Part model, mm, in its own coordinate system. Face numbers are marked on the shaded views. A direction names the side the tool comes from. Give positions to 0.01 mm unless a question says otherwise; leave off trailing zeros. Order: outer loops, then holes, each group sorted by start corner. A loop starts at its lowest first (then second) coordinate and runs counter-clockwise, first axis right, second up.
from build123d import *

# Parameters (mm, degrees)
SKETCH_7_W          = 180
SKETCH_7_H          = 128
EXTRUDE_1_DEPTH     = 2300
SKETCH_8_R          = 11.5
CUT_EXTRUDE_1_DEPTH = 16
SKETCH_9_R          = 11.5
CUT_EXTRUDE_2_DEPTH = 16


with BuildPart() as part:
    # 草图7 → 凸台-拉伸1 (new body)
    with BuildSketch(Plane(origin=(0, 0, 0), x_dir=(0, 0, -1), z_dir=(1, 0, 0))):
        Polygon((-315, 16), (-315, 0), (315, 0), (315, 16), (106, 16), (106, 144), (150, 144), (150, 160), (-150, 160), (-150, 144), (-106, 144), (-106, 16), align=None)
        with Locations((0, 80)):
            Rectangle(SKETCH_7_W, SKETCH_7_H, mode=Mode.SUBTRACT)
    extrude(amount=EXTRUDE_1_DEPTH)

    # 草图8 → 切除-拉伸1 (cut)
    with BuildSketch(Plane(origin=(0, 160, 0), x_dir=(1, 0, 0), z_dir=(0, 1, 0))):
        with Locations(Location((462.5, 62.5, 0), (0, 0, 270))):
            Circle(SKETCH_8_R)
        with Locations(Location((587.5, 62.5, 0), (0, 0, 270))):
            Circle(SKETCH_8_R)
        with Locations(Location((462.5, -62.5, 0), (0, 0, 270))):
            Circle(SKETCH_8_R)
        with Locations(Location((587.5, -62.5, 0), (0, 0, 270))):
            Circle(SKETCH_8_R)
        with Locations(Location((1712.5, 62.5, 0), (0, 0, 270))):
            Circle(SKETCH_8_R)
        with Locations(Location((1837.5, 62.5, 0), (0, 0, 270))):
            Circle(SKETCH_8_R)
        with Locations(Location((1712.5, -62.5, 0), (0, 0, 270))):
            Circle(SKETCH_8_R)
        with Locations(Location((1837.5, -62.5, 0), (0, 0, 270))):
            Circle(SKETCH_8_R)
    extrude(amount=-CUT_EXTRUDE_1_DEPTH, mode=Mode.SUBTRACT)

    # 草图9 → 切除-拉伸2 (cut)
    with BuildSketch(Plane.XZ):
        with Locations(Location((110, 260, 0), (0, 0, 270))):
            Circle(SKETCH_9_R)
        with Locations(Location((190, 260, 0), (0, 0, 270))):
            Circle(SKETCH_9_R)
        with Locations(Location((410, 260, 0), (0, 0, 270))):
            Circle(SKETCH_9_R)
        with Locations(Location((490, 260, 0), (0, 0, 270))):
            Circle(SKETCH_9_R)
        with Locations(Location((710, 260, 0), (0, 0, 270))):
            Circle(SKETCH_9_R)
        with Locations(Location((790, 260, 0), (0, 0, 270))):
            Circle(SKETCH_9_R)
        with Locations(Location((1110, 260, 0), (0, 0, 270))):
            Circle(SKETCH_9_R)
        with Locations(Location((1190, 260, 0), (0, 0, 270))):
            Circle(SKETCH_9_R)
        with Locations(Location((1510, 260, 0), (0, 0, 270))):
            Circle(SKETCH_9_R)
        with Locations(Location((1590, 260, 0), (0, 0, 270))):
            Circle(SKETCH_9_R)
        with Locations(Location((1810, 260, 0), (0, 0, 270))):
            Circle(SKETCH_9_R)
        with Locations(Location((1890, 260, 0), (0, 0, 270))):
            Circle(SKETCH_9_R)
        with Locations(Location((110, 180, 0), (0, 0, 270))):
            Circle(SKETCH_9_R)
        with Locations(Location((190, 180, 0), (0, 0, 270))):
            Circle(SKETCH_9_R)
        with Locations(Location((410, 180, 0), (0, 0, 270))):
            Circle(SKETCH_9_R)
        with Locations(Location((490, 180, 0), (0, 0, 270))):
            Circle(SKETCH_9_R)
        with Locations(Location((710, 180, 0), (0, 0, 270))):
            Circle(SKETCH_9_R)
        with Locations(Location((790, 180, 0), (0, 0, 270))):
            Circle(SKETCH_9_R)
        with Locations(Location((1110, 180, 0), (0, 0, 270))):
            Circle(SKETCH_9_R)
        with Locations(Location((1190, 180, 0), (0, 0, 270))):
            Circle(SKETCH_9_R)
        with Locations(Location((1510, 180, 0), (0, 0, 270))):
            Circle(SKETCH_9_R)
        with Locations(Location((1590, 180, 0), (0, 0, 270))):
            Circle(SKETCH_9_R)
        with Locations(Location((1810, 180, 0), (0, 0, 270))):
            Circle(SKETCH_9_R)
        with Locations(Location((1890, 180, 0), (0, 0, 270))):
            Circle(SKETCH_9_R)
        with Locations(Location((110, -140, 0), (0, 0, 270))):
            Circle(SKETCH_9_R)
        with Locations(Location((190, -140, 0), (0, 0, 270))):
            Circle(SKETCH_9_R)
        with Locations(Location((410, -140, 0), (0, 0, 270))):
            Circle(SKETCH_9_R)
        with Locations(Location((490, -140, 0), (0, 0, 270))):
            Circle(SKETCH_9_R)
        with Locations(Location((710, -140, 0), (0, 0, 270))):
            Circle(SKETCH_9_R)
        with Locations(Location((790, -140, 0), (0, 0, 270))):
            Circle(SKETCH_9_R)
        with Locations(Location((1110, -140, 0), (0, 0, 270))):
            Circle(SKETCH_9_R)
        with Locations(Location((1190, -140, 0), (0, 0, 270))):
            Circle(SKETCH_9_R)
        with Locations(Location((1510, -140, 0), (0, 0, 270))):
            Circle(SKETCH_9_R)
        with Locations(Location((1590, -140, 0), (0, 0, 270))):
            Circle(SKETCH_9_R)
        with Locations(Location((1810, -140, 0), (0, 0, 270))):
            Circle(SKETCH_9_R)
        with Locations(Location((1890, -140, 0), (0, 0, 270))):
            Circle(SKETCH_9_R)
        with Locations(Location((110, -220, 0), (0, 0, 270))):
            Circle(SKETCH_9_R)
        with Locations(Location((190, -220, 0), (0, 0, 270))):
            Circle(SKETCH_9_R)
        with Locations(Location((410, -220, 0), (0, 0, 270))):
            Circle(SKETCH_9_R)
        with Locations(Location((490, -220, 0), (0, 0, 270))):
            Circle(SKETCH_9_R)
        with Locations(Location((710, -220, 0), (0, 0, 270))):
            Circle(SKETCH_9_R)
        with Locations(Location((790, -220, 0), (0, 0, 270))):
            Circle(SKETCH_9_R)
        with Locations(Location((1110, -220, 0), (0, 0, 270))):
            Circle(SKETCH_9_R)
        with Locations(Location((1190, -220, 0), (0, 0, 270))):
            Circle(SKETCH_9_R)
        with Locations(Location((1510, -220, 0), (0, 0, 270))):
            Circle(SKETCH_9_R)
        with Locations(Location((1590, -220, 0), (0, 0, 270))):
            Circle(SKETCH_9_R)
        with Locations(Location((1810, -220, 0), (0, 0, 270))):
            Circle(SKETCH_9_R)
        with Locations(Location((1890, -220, 0), (0, 0, 270))):
            Circle(SKETCH_9_R)
        with Locations(Location((2110, 260, 0), (0, 0, 270))):
            Circle(SKETCH_9_R)
        with Locations(Location((2190, 260, 0), (0, 0, 270))):
            Circle(SKETCH_9_R)
        with Locations(Location((2110, 180, 0), (0, 0, 270))):
            Circle(SKETCH_9_R)
        with Locations(Location((2190, 180, 0), (0, 0, 270))):
            Circle(SKETCH_9_R)
        with Locations(Location((2110, -140, 0), (0, 0, 270))):
            Circle(SKETCH_9_R)
        with Locations(Location((2190, -140, 0), (0, 0, 270))):
            Circle(SKETCH_9_R)
        with Locations(Location((2110, -220, 0), (0, 0, 270))):
            Circle(SKETCH_9_R)
        with Locations(Location((2190, -220, 0), (0, 0, 270))):
            Circle(SKETCH_9_R)
    extrude(amount=-CUT_EXTRUDE_2_DEPTH, mode=Mode.SUBTRACT)


solid = part.part
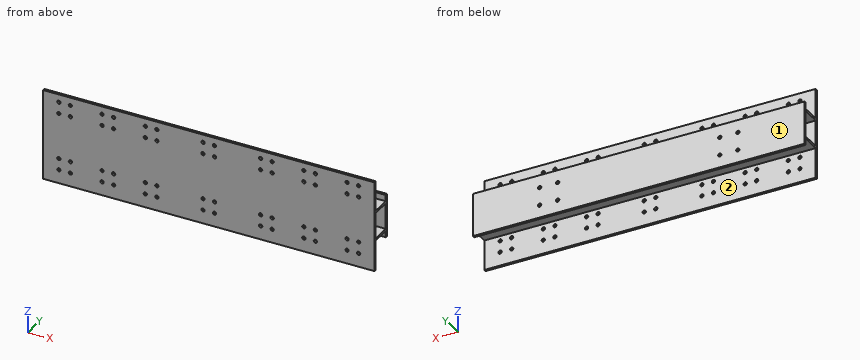
Item 1: Drill centre lines: probe 1 along Z at (x, y) = (1590, 8); probe 2 along Y at (x, z) = (1551, -135); probe 3 along Z at (x, y) = (2133.5, 43). Where is each one in solid material? Low to high.
Item 2: Drop flat-ended pins along their axis: P1, Ø10, axis at x = 972.5, y = 59, coming from the +Z side; P2, Ø12, axis at x = 829.5, y = 109, coming from the -Z side; P3, Ø20.5, axis at x = 490, z = 180, coming from the -Y side; P4, Ø14, axis at x = 1712.5, z = 62.5, coming from the +Y side. Give the stop position or say it passes through.
Item 3: Band-saw the part on A-A on y = 103. List the corners of the cut face in (x, z), plus the area to 3 significant figures.
Item 4: Band-saw the part on C-C on x = 994. List the corners of the cut face in (y, z), plus the area to 3 significant figures.
Item 5: Band-saw the part on B-B on z = -9. List the corners of the cut face in (x, y).
Item 6: Which spindle directions (+Z, -Z, +X, -X, +Y, -Y) get a long thin tool onto all of the face, cutting with end or side? Do the marked faces 1 and 2. Say none if no direction does.
Working result:
1. probe 1: z = -315 to -231.5, -208.5 to -151.5, -128.5 to 168.5, 191.5 to 248.5, 271.5 to 315
1. probe 2: y = 0 to 16, 144 to 160
1. probe 3: z = -106 to -90, 90 to 106
2. P1: stops at z = 106
2. P2: stops at z = -106
2. P3: passes through
2. P4: stops at y = 16
3. outline: (0, -106) - (2300, -106) - (2300, -90) - (0, -90) - close; (0, 90) - (2300, 90) - (2300, 106) - (0, 106) - close
3. area: 73,600 mm2
4. outline: (0, -315) - (16, -315) - (16, -106) - (144, -106) - (144, -150) - (160, -150) - (160, 150) - (144, 150) - (144, 106) - (16, 106) - (16, 315) - (0, 315) - close; hole (16, -90) - (144, -90) - (144, 90) - (16, 90) - close
4. area: 19,000 mm2
5. outline: (0, 0) - (2300, 0) - (2300, 16) - (0, 16) - close; (0, 144) - (2300, 144) - (2300, 160) - (0, 160) - close
6. face 1: +Z, -Z, +X, -X, +Y
6. face 2: -Z, +X, -X
